```python
from build123d import *

# Parameters (mm, degrees)
SKETCH1_R           = 101.6
BOSS_EXTRUDE1_DEPTH = 76.2
SKETCH2_R           = 88.9
CUT_EXTRUDE1_DEPTH  = 63.5
SKETCH3_R           = 12.7
SKETCH3_R_2         = 9.525
BOSS_EXTRUDE2_DEPTH = 25.4


with BuildPart() as part:
    # Sketch1 → Boss-Extrude1 (new body)
    with BuildSketch(Plane(origin=(0, 0, 0), x_dir=(1, 0, 0), z_dir=(0, 1, 0))):
        Circle(SKETCH1_R)
    extrude(amount=BOSS_EXTRUDE1_DEPTH)

    # Sketch2 → Cut-Extrude1 (cut)
    with BuildSketch(Plane(origin=(0, 76.2, 0), x_dir=(1, 0, 0), z_dir=(0, 1, 0))):
        Circle(SKETCH2_R)
    extrude(amount=-CUT_EXTRUDE1_DEPTH, mode=Mode.SUBTRACT)

    # Sketch3 → Boss-Extrude2 (add)
    with BuildSketch(Plane.XZ):
        Circle(SKETCH3_R)
        Circle(SKETCH3_R_2, mode=Mode.SUBTRACT)
    extrude(amount=BOSS_EXTRUDE2_DEPTH)


solid = part.part
```
Check sheet for the modelled part. Datum: model origin and axes. Units: mm. A direction names the side the tool comes from. Give positions to 0.01 mm unless a question says otherwise; leave off trailing zeros. Write each loop counter-clockwise with the first axis right and the second up, starting at its lowest first coordinate (ties: lowest second). Pieces come first, ordered by that corner, then holes. Notation, with made-up numbers: (9.5, 62) -> (35.5, 62) arc R16 cw to (35.5, 68) -> close; hole circle Ø4 at (81, 25.25). An arc over 180 degrees is marked (long way). Use CSV: the item, a comma, the result in double quotes. Start each with the question number.
Q1. Tool access check on faces 1 (the flat face through (0, 0, 0)), 2 (the flat face through (5, -25.4, 9)), 3 (the cylindrical face through (84.795, 44.894, -26.703)). Record the directions out of +Z, -Z, +X, -X, +Y, -Y that give a thin tool (end or side, any length) a straight path to the whole face; none if there is none.
Q2. Cross-section at D-D on y = -17.5. Enter the section's corners in (x, z) (3 decimals).
Q3. Scan lines: line 1 along X through (y, z) = (40, 0); line 2 along Y through (x, z) = (13, -13). Record each from-to range of solid material in increasing order.
Q4. Release check for a two-part mould opening along X. For faces 4 (the flat face through (0, 76.2, 90)), 5 (the cylindrical face through (-22.025, 37.567, 99.184)), 6 (the cylindrical face through (-7.559, -12.522, -5.796)) record: +X half, -X half, draft (parallel to the pull), parting line (faces both ways), or undercut.
Q5. Cross-section at C-C on y = 32.5. Enter the section's corners in (x, z).
Q6. Cross-section at B-B on x = 0. Enter the section's corners in (y, z) (3 decimals).
Q7. Cross-section at A-A on z = 0. Enter the section's corners in (x, y) (3 decimals).
Q8. Depth check by flat-ended pin: P1, Ø8, axis at y = 31.5, z = -65.5, coming from the +X side; P2, Ø2, axis at x = -78, y = 61.5, coming from the -Z side; P3, Ø8, axis at x = -32, y = 37.5, coming from the -Z side; P4, Ø25, axis at x = 0, z = 0, coming from the -Y side. Enter the tip coordinate at first touch or a pass-through.
Working result:
1,face 1,"-Y"
1,face 2,"+Z, -Z, +X, -X, -Y"
1,face 3,"+Y"
2,outline,"circle Ø25.4 at (0, 0); hole circle Ø19.05 at (0, 0)"
3,line 1,"x = -101.6 to -88.9, 88.9 to 101.6"
3,line 2,"y = 0 to 12.7"
4,face 4,"draft"
4,face 5,"parting line"
4,face 6,"undercut"
5,outline,"circle Ø203.2 at (0, 0); hole circle Ø177.8 at (0, 0)"
6,outline,"(-25.4, -12.7) -> (0, -12.7) -> (0, -101.6) -> (76.2, -101.6) -> (76.2, -88.9) -> (12.7, -88.9) -> (12.7, 88.9) -> (76.2, 88.9) -> (76.2, 101.6) -> (0, 101.6) -> (0, 12.7) -> (-25.4, 12.7) -> (-25.4, 9.525) -> (0, 9.525) -> (0, -9.525) -> (-25.4, -9.525) -> close"
7,outline,"(-101.6, 0) -> (-12.7, 0) -> (-12.7, -25.4) -> (-9.525, -25.4) -> (-9.525, 0) -> (9.525, 0) -> (9.525, -25.4) -> (12.7, -25.4) -> (12.7, 0) -> (101.6, 0) -> (101.6, 76.2) -> (88.9, 76.2) -> (88.9, 12.7) -> (-88.9, 12.7) -> (-88.9, 76.2) -> (-101.6, 76.2) -> close"
8,P1,"stops at x = 80.87"
8,P2,"stops at z = -66.28"
8,P3,"stops at z = -97.67"
8,P4,"stops at y = -25.4"
